Geometry check sheet. Reference: the model listing, model coordinates, mm. A direction names the side the tool comes from. Round coordinates to 2 decimals unless told otherwise and drop trailing zeros. Order: outer loops, then holes, each group sorted by start corner. A loop starts at its lowest first (then second) coordinate and runs counter-clockwise, first axis right, second up. Notation, with made-up numbers: (40.5, 2) -> (48.5, 2) arc R30 ccw to (48.5, 38) -> close; hole circle Ø8 at (77, 62.5). An arc over 180 degrees is marked (long way). Answer as a JSON object with one key per item and string values. Group by question number.
from build123d import *

# Parameters (mm, degrees)
SKETCH1_W           = 32.9
SKETCH1_H           = 22.4
BOSS_EXTRUDE1_DEPTH = 5
SKETCH2_R           = 1.2
SKETCH2_W           = 22.9
SKETCH2_H           = 12.4
CUT_EXTRUDE2_DEPTH  = 5
SKETCH3_W           = 22.996888994
SKETCH3_H           = 5
BOSS_EXTRUDE2_DEPTH = 12.3
SKETCH4_R           = 1.2
CUT_EXTRUDE3_DEPTH  = 5
SKETCH6_W           = 5
SKETCH6_H           = 5
SKETCH6_W_2         = 4.903111006
BOSS_EXTRUDE3_DEPTH = 12.3
SKETCH8_W           = 17.3
SKETCH8_H           = 4.998204887
BOSS_EXTRUDE4_DEPTH = 3.1
SKETCH9_W           = 17.3
SKETCH9_H           = 5
BOSS_EXTRUDE5_DEPTH = 3.1
SKETCH18_W          = 5
SKETCH18_H          = 12.4
BOSS_EXTRUDE7_DEPTH = 30
SKETCH19_R          = 4.5
CUT_EXTRUDE6_DEPTH  = 30
SKETCH20_R          = 4.5
CUT_EXTRUDE7_DEPTH  = 30
SKETCH10_W          = 5
SKETCH10_H          = 12.4
BOSS_EXTRUDE6_DEPTH = 30
SKETCH21_R          = 4.5
CUT_EXTRUDE8_DEPTH  = 10
SKETCH22_R          = 4.5
CUT_EXTRUDE9_DEPTH  = 10
CUT_EXTRUDE10_DEPTH = 3
SKETCH25_W          = 2.45
SKETCH25_H          = 22.4
SKETCH25_W_2        = 0.55
CUT_EXTRUDE11_DEPTH = 40.1


with BuildPart() as part:
    # Sketch1 → Boss-Extrude1 (new body)
    with BuildSketch(Plane.XY):
        Rectangle(SKETCH1_W, SKETCH1_H)
    extrude(amount=BOSS_EXTRUDE1_DEPTH)

    # Sketch2 → Cut-Extrude2 (cut)
    with BuildSketch(Plane.XY.offset(5)):
        with Locations((13.8, 0)):
            Circle(SKETCH2_R)
        with Locations((-13.8, 0)):
            Circle(SKETCH2_R)
        Rectangle(SKETCH2_W, SKETCH2_H)
    extrude(amount=-CUT_EXTRUDE2_DEPTH, mode=Mode.SUBTRACT)

    # Sketch3 → Boss-Extrude2 (add)
    with BuildSketch(Plane.XY.offset(5)):
        with Locations((0.048444497, 8.7)):
            Rectangle(SKETCH3_W, SKETCH3_H)
        with Locations((0.048444497, -8.7)):
            Rectangle(SKETCH3_W, SKETCH3_H)
    extrude(amount=BOSS_EXTRUDE2_DEPTH)

    # Sketch4 → Cut-Extrude3 (cut)
    with BuildSketch(Plane.XY.offset(17.3)):
        with Locations((0.048444497, 8.7)):
            Circle(SKETCH4_R)
        with Locations((0.048444497, -8.7)):
            Circle(SKETCH4_R)
    extrude(amount=-CUT_EXTRUDE3_DEPTH, mode=Mode.SUBTRACT)

    # Sketch6 → Boss-Extrude3 (add)
    with BuildSketch(Plane.XY.offset(5)):
        with Locations((-13.95, -8.7)):
            Rectangle(SKETCH6_W, SKETCH6_H)
        with Locations((13.998444497, -8.7)):
            Rectangle(SKETCH6_W_2, SKETCH6_H)
    extrude(amount=BOSS_EXTRUDE3_DEPTH)

    # Sketch8 → Boss-Extrude4 (add)
    with BuildSketch(Plane(origin=(16.45, 0, 0), x_dir=(0, 0, -1), z_dir=(1, 0, 0))):
        with Locations((-8.65, -8.700897557)):
            Rectangle(SKETCH8_W, SKETCH8_H)
    extrude(amount=BOSS_EXTRUDE4_DEPTH)

    # Sketch9 → Boss-Extrude5 (add)
    with BuildSketch(Plane.ZY.offset(16.45)):
        with Locations((8.65, -8.7)):
            Rectangle(SKETCH9_W, SKETCH9_H)
    extrude(amount=BOSS_EXTRUDE5_DEPTH)

    # Sketch18 → Boss-Extrude7 (add)
    with BuildSketch(Plane.XZ.offset(11.2)):
        with Locations((-17.05, 8.65)):
            Rectangle(SKETCH18_W, SKETCH18_H)
        with Locations((17.05, 8.65)):
            Rectangle(SKETCH18_W, SKETCH18_H)
    extrude(amount=BOSS_EXTRUDE7_DEPTH)

    # Sketch19 → Cut-Extrude6 (cut)
    with BuildSketch(Plane.ZY.offset(19.55)):
        with Locations((8.65, -34.8)):
            Circle(SKETCH19_R)
    extrude(amount=-CUT_EXTRUDE6_DEPTH, mode=Mode.SUBTRACT)

    # Sketch20 → Cut-Extrude7 (cut)
    with BuildSketch(Plane(origin=(19.55, 0, 0), x_dir=(0, 0, -1), z_dir=(1, 0, 0))):
        with Locations((-8.65, -34.8)):
            Circle(SKETCH20_R)
    extrude(amount=-CUT_EXTRUDE7_DEPTH, mode=Mode.SUBTRACT)

    # Sketch10 → Boss-Extrude6 (add)
    with BuildSketch(Plane.XZ.offset(11.2)):
        with Locations((17.05, 8.65)):
            Rectangle(SKETCH10_W, SKETCH10_H)
        with Locations((-17.05, 8.65)):
            Rectangle(SKETCH10_W, SKETCH10_H)
    extrude(amount=BOSS_EXTRUDE6_DEPTH)

    # Sketch21 → Cut-Extrude8 (cut)
    with BuildSketch(Plane(origin=(19.55, 0, 0), x_dir=(0, 0, -1), z_dir=(1, 0, 0))):
        with Locations((-8.65, -34.8)):
            Circle(SKETCH21_R)
    extrude(amount=-CUT_EXTRUDE8_DEPTH, mode=Mode.SUBTRACT)

    # Sketch22 → Cut-Extrude9 (cut)
    with BuildSketch(Plane(origin=(-14.55, 0, 0), x_dir=(0, 0, -1), z_dir=(1, 0, 0))):
        with Locations((-8.65, -34.8)):
            Circle(SKETCH22_R)
    extrude(amount=-CUT_EXTRUDE9_DEPTH, mode=Mode.SUBTRACT)

    # Sketch23 → Cut-Extrude10 (cut)
    with BuildSketch(Plane.ZY.offset(19.55)):
        with BuildLine():
            Line((5.65, -22.3), (4.674239456, -32.692079676))
            ThreePointArc((4.674239456, -32.692079676), (8.65, -30.3), (12.625760544, -32.692079676))
            Line((12.625760544, -32.692079676), (11.65, -22.3))
            ThreePointArc((11.65, -22.3), (8.65, -19.3), (5.65, -22.3))
        make_face()
    extrude(amount=-CUT_EXTRUDE10_DEPTH, mode=Mode.SUBTRACT)

    # Sketch25 → Cut-Extrude11 (cut, through all)
    with BuildSketch(Plane.ZY.offset(19.55)):
        with Locations((16.075, 0)):
            Rectangle(SKETCH25_W, SKETCH25_H)
        with Locations((0.275, 0)):
            Rectangle(SKETCH25_W_2, SKETCH25_H)
    extrude(amount=-CUT_EXTRUDE11_DEPTH, mode=Mode.SUBTRACT)


solid = part.part
Item 1: Thickness scan on L1, parallel to Y at x = 6, z = 1.75; L2, parallel to Z at x = -17.85, y = -34.8; L3, parallel to X at y = -11.5, z = 8. Record the ranges inside material, lowest first.
Item 2: Depth check by flat-ended pin: pin 1 Ø2 at (y, z) = (-1, 1.5) entering from -X; pin 2 Ø2.5 at (x, y) = (-14, 3.5) entering from +Z; pin 3 Ø4 at (y, z) = (9.5, 12.5) entering from +X. Enter the tip coordinate at first touch or a pass-through.
Item 3: Sectioned sample at D-D, the plane y = -28.5. Enter the section's corners in (x, z), then the cut area to 3 significant figures.
Item 4: Set-up check for faces 1 (the flat face through (11.45, 0, 3)), 2 (the flat face through (11.547, 9, 10)), 3 (the flat face through (-16.55, -26, 9)), 4 (the cylindrical face through (-0.11, -7.51, 13.59)): record each of +Z, -Z, +X, -X, +Y, -Y from which the full face is reachable in a straight line by a thin tool's end or side.
Item 5: Sectioned sample at C-C, the plane y = 0. Enter the section's corners in (x, z), then the cut area to 3 significant figures.
Item 6: Mould release check, pull along Z, two halves, no side actions. Record for faces 5 (the flat face through (0, 9, 12.3)), 6 (the flat face through (-17, -41.2, 9)), 7 (the cylindrical face through (17.08, -31.76, 11.97)): pulls with the +Z half, pulls with the -Z half, needs draft (parallel to the pull), parting line crosses it, or undercut.
Item 7: Sectioned sample at A-A, the plane x = 13.8. Enter the section's corners in (y, z).
Item 8: Sectioned sample at B-B, the plane z = 8.65. Count the separate pieces of the cut face and the enclosed holes in it, then the cut area to 3 significant figures.
Result:
{
 "1": {"L1": "y = -11.2 to -6.2, 6.2 to 11.2", "L2": "z = 2.45 to 4.15, 13.15 to 14.85", "L3": "x = -19.55 to -14.55, 14.55 to 19.55"},
 "2": {"pin 1": "stops at x = -16.45", "pin 2": "stops at z = 5", "pin 3": "stops at x = 11.55"},
 "3": {"outline": "(-19.55, 2.45) -> (-14.55, 2.45) -> (-14.55, 14.85) -> (-19.55, 14.85) -> (-19.55, 12.23) -> (-16.55, 12.23) -> (-16.55, 5.07) -> (-19.55, 5.07) -> close; (14.55, 2.45) -> (19.55, 2.45) -> (19.55, 14.85) -> (14.55, 14.85) -> close", "area": "103 mm2"},
 "4": {"face 1": "+Z, -Z", "face 2": "+Z, +X, +Y", "face 3": "-X", "face 4": "+Z"},
 "5": {"outline": "(-16.45, 0.55) -> (-15, 0.55) -> (-15, 5) -> (-16.45, 5) -> close; (-12.6, 0.55) -> (-11.45, 0.55) -> (-11.45, 5) -> (-12.6, 5) -> close; (11.45, 0.55) -> (12.6, 0.55) -> (12.6, 5) -> (11.45, 5) -> close; (15, 0.55) -> (16.45, 0.55) -> (16.45, 5) -> (15, 5) -> close", "area": "23.1 mm2"},
 "6": {"face 5": "pulls with the +Z half", "face 6": "needs draft", "face 7": "undercut"},
 "7": {"outline": "(-11.2, 0.55) -> (-1.2, 0.55) -> (-1.2, 5) -> (-6.2, 5) -> (-6.2, 14.85) -> (-11.2, 14.85) -> close; (1.2, 0.55) -> (11.2, 0.55) -> (11.2, 5) -> (1.2, 5) -> close"},
 "8": {"separate pieces": "4", "enclosed holes": "0", "area": "487 mm2"}
}
